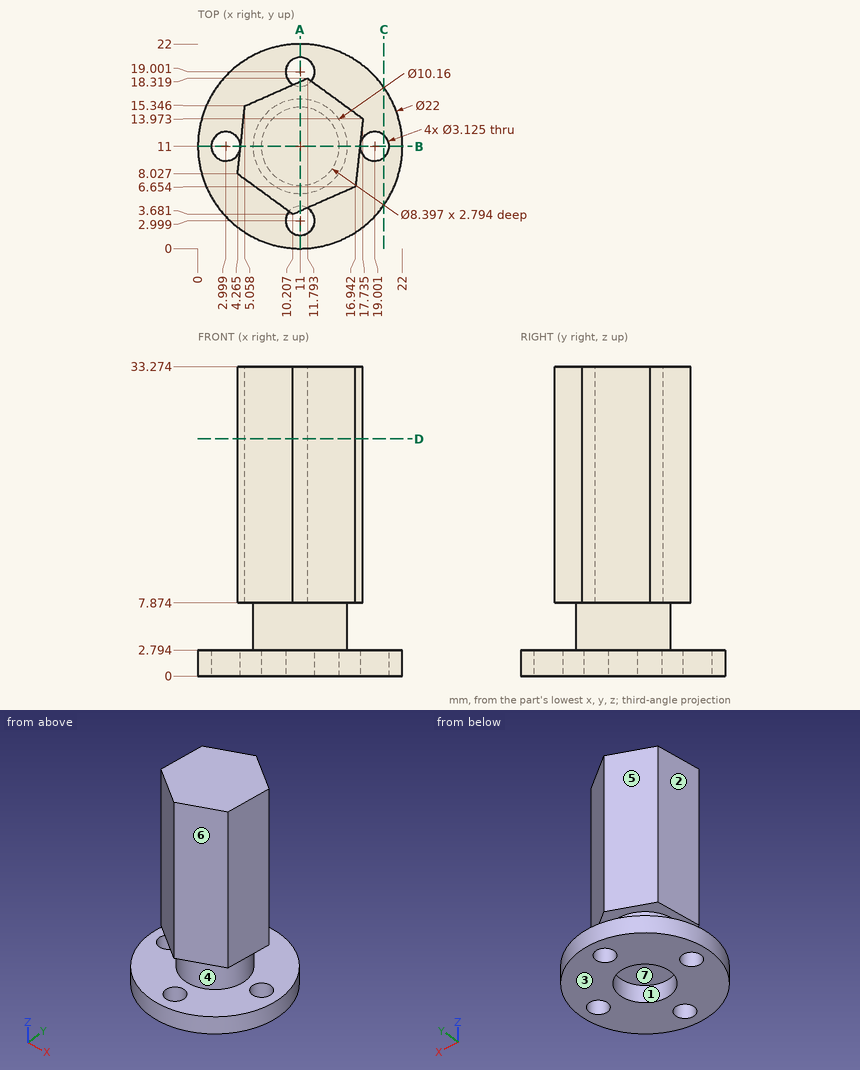
Design review of the part shown in the three views and the two pictorial views. Dimensions are in mm from the part's minimum x, y and z. A direction names the side the tool comes from. Round coordinates to 2 decimals unless told otherwise and drop trailing zeros. Write each loop counter-clockwise with the first axis right and the second up, starting at its lowest first coordinate (ties: lowest second). Pieces come first, ordered by that corner, then holes. Notation, with made-up numbers: (8, 21) -> (49, 21) arc R29 cw to (49, 44) -> close; hole circle Ø9 at (37, 55.5). An arc over 180 degrees is marked (long way). One line per question, with ' | ' between items. Start each with the question number.
1) Wall thickness on line 1 along Y through (x, z) = (11, 2.15); line 2 along Z through (x, y) = (16.25, 14); line 3 along Z through (x, y) = (9.5, 7.5): over which ranges is each line inside the solid? List them lowest first.
2) Add section D-D (z = 25.5). Write out the cut boundary in (x, y) (1 decimal).
3) Mouldability with a two-part tool opening along Y and no side actions: class the marked faces 1, 2 and 3 as +Y half, -Y half, draft (parallel to the pull), parting line (faces both ways), or undercut.
4) Add section C-C (x = 20). Write out the cut boundary in (y, z) (1 decimal).
5) Add section A-A (x = 11). Write out the cut boundary in (y, z).
6) For pin 1 Ø2 at (x, y) = (9.5, 10.5) entering from -Z; pin 2 Ø2.5 at (x, y) = (19.001, 11) entering from +Z; pin 3 Ø3 at (x, y) = (3, 12) entering from +Z; pin 4 Ø5 at (x, z) = (3.5, 28.5) entering from -Y, all flat-tipped, find the tip position at first contact; note any pin that passes through.
7) Add section B-B (y = 11). Write out the cut boundary in (x, z), and give its area (3 significant figures).
8) Machinability: for the marked faces 4, 5, 6 and 7, which of the approach directions +Z, -Z, +X, -X, +Y, -Y give a long, thin tool a straight path to every point of the face, cutting with its end or side? Answer none if there is none.
Reported:
1) line 1: y = 0 to 1.44, 4.56 to 6.8, 15.2 to 17.44, 20.56 to 22 | line 2: z = 0 to 2.79, 7.87 to 33.27 | line 3: z = 2.79 to 33.27
2) outline: (4.3, 8) -> (10.2, 3.7) -> (16.9, 6.7) -> (17.7, 14) -> (11.8, 18.3) -> (5.1, 15.3) -> close
3) face 1: undercut | face 2: +Y half | face 3: draft
4) outline: (4.7, 0) -> (9.8, 0) -> (9.8, 2.8) -> (4.7, 2.8) -> close; (12.2, 0) -> (17.3, 0) -> (17.3, 2.8) -> (12.2, 2.8) -> close
5) outline: (0, 0) -> (1.44, 0) -> (1.44, 2.79) -> (0, 2.79) -> close; (4.03, 7.87) -> (5.92, 7.87) -> (5.92, 2.79) -> (4.56, 2.79) -> (4.56, 0) -> (6.8, 0) -> (6.8, 2.79) -> (15.2, 2.79) -> (15.2, 0) -> (17.44, 0) -> (17.44, 2.79) -> (16.08, 2.79) -> (16.08, 7.87) -> (17.97, 7.87) -> (17.97, 33.27) -> (4.03, 33.27) -> close; (20.56, 0) -> (22, 0) -> (22, 2.79) -> (20.56, 2.79) -> close
6) pin 1: stops at z = 2.79 | pin 2: passes through | pin 3: stops at z = 2.79 | pin 4: stops at y = 6.76
7) outline: (0, 0) -> (1.44, 0) -> (1.44, 2.79) -> (0, 2.79) -> close; (4.56, 0) -> (6.8, 0) -> (6.8, 2.79) -> (15.2, 2.79) -> (15.2, 0) -> (17.44, 0) -> (17.44, 2.79) -> (16.08, 2.79) -> (16.08, 7.87) -> (17.41, 7.87) -> (17.41, 33.27) -> (4.59, 33.27) -> (4.59, 7.87) -> (5.92, 7.87) -> (5.92, 2.79) -> (4.56, 2.79) -> close; (20.56, 0) -> (22, 0) -> (22, 2.79) -> (20.56, 2.79) -> close | area: 398 mm²
8) face 4: none | face 5: +Z, -X, +Y | face 6: +Z, +X, -Y | face 7: -Z
